Verification items for the finished model (mm, model axes). A direction names the side the tool comes from. Round coordinates to 2 decimals unless told otherwise and drop trailing zeros. Write each loop counter-clockwise with the first axis right and the second up, starting at its lowest first coordinate (ties: lowest second). Pieces come first, ordered by that corner, then holes.
from build123d import *

# Parameters (mm, degrees)
F0_R     = 50.8
F1_DEPTH = 6.35
F3_DEPTH = 3.175


with BuildPart() as f1:
    # F0 (on Top) → F1 (new body)
    with BuildSketch(Plane.XY):
        Circle(F0_R)
    extrude(amount=F1_DEPTH)

    # F2 (on face) → F3 (cut)
    with BuildSketch(Plane.XY.offset(6.35)):
        with BuildLine():
            ThreePointArc((-2.023529, -34.533925), (-1.777175, -28.603001), (0, -22.939239))
            ThreePointArc((0, -22.939239), (1.777175, -28.603001), (2.023529, -34.533925))
            Line((2.023529, -34.533925), (5.974615, -34.669533))
            ThreePointArc((5.974615, -34.669533), (7.104242, -28.355202), (9.302336, -22.328991))
            ThreePointArc((9.302336, -22.328991), (10.967211, -23.551895), (11.607712, -25.515836))
            Line((11.607712, -25.515836), (11.539907, -35.957832))
            ThreePointArc((11.539907, -35.957832), (14.380524, -35.985773), (16.96432, -34.805145))
            ThreePointArc((16.96432, -34.805145), (18.085967, -26.770231), (16.96432, -18.735318))
            ThreePointArc((16.96432, -18.735318), (16.7578, -14.870423), (16.96432, -11.005528))
            ThreePointArc((16.96432, -11.005528), (17.869083, -9.379184), (19.066282, -7.954295))
            ThreePointArc((19.066282, -7.954295), (24.814172, -7.002965), (30.554628, -6.007752))
            ThreePointArc((30.554628, -6.007752), (36.833108, -2.099002), (39.505046, 4.797257))
            ThreePointArc((39.505046, 4.797257), (37.343339, 20.639318), (29.19136, 34.393921))
            ThreePointArc((29.19136, 34.393921), (27.094397, 36.509907), (24.600387, 38.139191))
            Line((24.600387, 38.139191), (22.805873, 29.13427))
            Line((22.805873, 29.13427), (11.843341, 26.337616))
            ThreePointArc((11.843341, 26.337616), (18.827134, 32.024386), (21.200456, 40.712312))
            ThreePointArc((21.200456, 40.712312), (11.071856, 45.336169), (0, 46.512008))
            ThreePointArc((0, 46.512008), (-11.071856, 45.336169), (-21.200456, 40.712312))
            ThreePointArc((-21.200456, 40.712312), (-18.827134, 32.024386), (-11.843341, 26.337616))
            Line((-11.843341, 26.337616), (-22.805873, 29.13427))
            Line((-22.805873, 29.13427), (-24.600387, 38.139191))
            ThreePointArc((-24.600387, 38.139191), (-27.094397, 36.509907), (-29.19136, 34.393921))
            ThreePointArc((-29.19136, 34.393921), (-37.343339, 20.639318), (-39.505046, 4.797257))
            ThreePointArc((-39.505046, 4.797257), (-36.833108, -2.099002), (-30.554628, -6.007752))
            ThreePointArc((-30.554628, -6.007752), (-24.814172, -7.002965), (-19.066282, -7.954295))
            ThreePointArc((-19.066282, -7.954295), (-17.869083, -9.379184), (-16.96432, -11.005528))
            ThreePointArc((-16.96432, -11.005528), (-16.7578, -14.870423), (-16.96432, -18.735318))
            ThreePointArc((-16.96432, -18.735318), (-18.085967, -26.770231), (-16.96432, -34.805145))
            ThreePointArc((-16.96432, -34.805145), (-14.380524, -35.985773), (-11.539907, -35.957832))
            Line((-11.539907, -35.957832), (-11.607712, -25.515836))
            ThreePointArc((-11.607712, -25.515836), (-10.967211, -23.551895), (-9.302336, -22.328991))
            ThreePointArc((-9.302336, -22.328991), (-7.104242, -28.355202), (-5.974615, -34.669533))
            Line((-5.974615, -34.669533), (-2.023529, -34.533925))
        make_face()
        with BuildLine():
            ThreePointArc((-2.023529, 2.753796), (-0.940643, -1.901231), (-0.975282, -6.680429))
            ThreePointArc((-0.975282, -6.680429), (-0.824525, -9.996426), (0, -13.211815))
            ThreePointArc((0, -13.211815), (0.824525, -9.996426), (0.975282, -6.680429))
            ThreePointArc((0.975282, -6.680429), (0.940643, -1.901231), (2.023529, 2.753796))
            ThreePointArc((2.023529, 2.753796), (5.148448, -3.217282), (5.974615, -9.905805))
            ThreePointArc((5.974615, -9.905805), (5.866823, -13.807024), (5.168271, -17.646706))
            ThreePointArc((5.168271, -17.646706), (2.647612, -16.831793), (0, -16.920999))
            ThreePointArc((0, -16.920999), (-2.647612, -16.831793), (-5.168271, -17.646706))
            ThreePointArc((-5.168271, -17.646706), (-5.866823, -13.807024), (-5.974615, -9.905805))
            ThreePointArc((-5.974615, -9.905805), (-5.148448, -3.217282), (-2.023529, 2.753796))
        make_face(mode=Mode.SUBTRACT)
        with BuildLine():
            ThreePointArc((-26.502606, 0), (-32.082928, 3.574671), (-32.482646, 10.189692))
            ThreePointArc((-32.482646, 10.189692), (-25.002638, 17.61113), (-14.542522, 16.340593))
            ThreePointArc((-14.542522, 16.340593), (-9.236558, 11.068946), (-6.683039, 4.038792))
            ThreePointArc((-6.683039, 4.038792), (-8.309473, 1.28099), (-11.243723, 0))
            ThreePointArc((-11.243723, 0), (-18.873164, -0.655974), (-26.502606, 0))
        make_face(mode=Mode.SUBTRACT)
        with BuildLine():
            ThreePointArc((11.243723, 0), (8.309473, 1.28099), (6.683039, 4.038792))
            ThreePointArc((6.683039, 4.038792), (9.236558, 11.068946), (14.542522, 16.340593))
            ThreePointArc((14.542522, 16.340593), (25.002638, 17.61113), (32.482646, 10.189692))
            ThreePointArc((32.482646, 10.189692), (32.082928, 3.574671), (26.502606, 0))
            ThreePointArc((26.502606, 0), (18.873164, -0.655974), (11.243723, 0))
        make_face(mode=Mode.SUBTRACT)
    extrude(amount=-F3_DEPTH, mode=Mode.SUBTRACT)


solid = f1.part
Q1. Sectioned sample at A-A (z = 4.5). Give the number of separate pieces and of enclosed holes in the cut face, plus the area to 3 significant figures.
Recorded:
separate pieces: 4
enclosed holes: 1
area: 4,800 mm2
Q2. Depth check by flat-ended pin: P1, Ø4, axis at x = -6, y = 38.5, coming from the -Z side; P2, Ø3, axis at x = -12, y = -19.5, coming from the +Z side (3 decimals); P3, Ø2, axis at y = -1.5, z = 5.5, coming from the -X side. Enter the tip coordinate at first touch or a pass-through.
Recorded:
P1: stops at z = 0
P2: stops at z = 3.175
P3: stops at x = -50.8
Q3. Material ranges on line 1 along Y through (x, z) = (-27, 3.75); line 2 along X through (y, z) = (-4, 5.25); line 3 along Y through (x, z) = (30, 4.25), recorded low to high.
Recorded:
line 1: y = -43.03 to -6.63, 0.07 to 16.72, 36.59 to 43.03
line 2: x = -50.64 to -34.84, -5.37 to -0.82, 0.82 to 5.37, 34.84 to 50.64
line 3: y = -41 to -6.11, 1.31 to 14.34, 33.47 to 41
Q4. Tool access check on faces 3 (the flat face through (-20, 9, 6.35)), 4 (the cylindrical face through (9.18, 10.98, 4.78)). Record the directions out of +Z, -Z, +X, -X, +Y, -Y that give a thin tool (end or side, any length) a straight path to the whole face; none if there is none.
Recorded:
face 3: +Z, +X, -X, +Y, -Y
face 4: +Z
Q5. Sectioned sample at B-B (x = -36). Enter the section's corners in (y, z) (3 decimals), plus the area to 3 significant figures.
Recorded:
outline: (-35.842, 0) - (35.842, 0) - (35.842, 6.35) - (24, 6.35) - (24, 3.175) - (-3.003, 3.175) - (-3.003, 6.35) - (-35.842, 6.35) - close
area: 369 mm2
Q6. Release check for a two-part mould opening along X. For faces 1 (the cylindrical face through (-11, -23.6, 4.8)), 2 (the flat face through (22, -11, 6.35)) record: released by +X, released by -X, zero draft, split by the parting line, or undercut.
Recorded:
face 1: undercut
face 2: zero draft
Q7. Sectioned sample at D-D (x = 41). Enter the section's corners in (y, z).
Recorded:
outline: (-29.99, 0) - (29.99, 0) - (29.99, 6.35) - (-29.99, 6.35) - close
Q8. Sectioned sample at C-C (y = 13.5). Enter the section's corners in (x, z) (3 decimals).
Recorded:
outline: (-48.973, 0) - (48.973, 0) - (48.973, 6.35) - (39.12, 6.35) - (39.12, 3.175) - (30.698, 3.175) - (30.698, 6.35) - (11.117, 6.35) - (11.117, 3.175) - (-11.117, 3.175) - (-11.117, 6.35) - (-30.698, 6.35) - (-30.698, 3.175) - (-39.12, 3.175) - (-39.12, 6.35) - (-48.973, 6.35) - close
